Can you work these out from the drawing? Everything is in mm from the part's minimum corner. A direction names the side the tool comes from. Round coordinates to 2 decimals unless told otherwise and drop trailing zeros. Loops run counter-clockwise (first coordinate to the right, second up) from the corner with the lowest first, then second, coordinate; pieces in that order, holes last. Notation, with made-up numbers: (21.25, 18) -> (58.25, 18) arc R32 cw to (58.25, 55) -> close; hole circle Ø11 at (17.25, -13.75). An arc over 180 degrees is marked (long way). One line per item, written item: value.
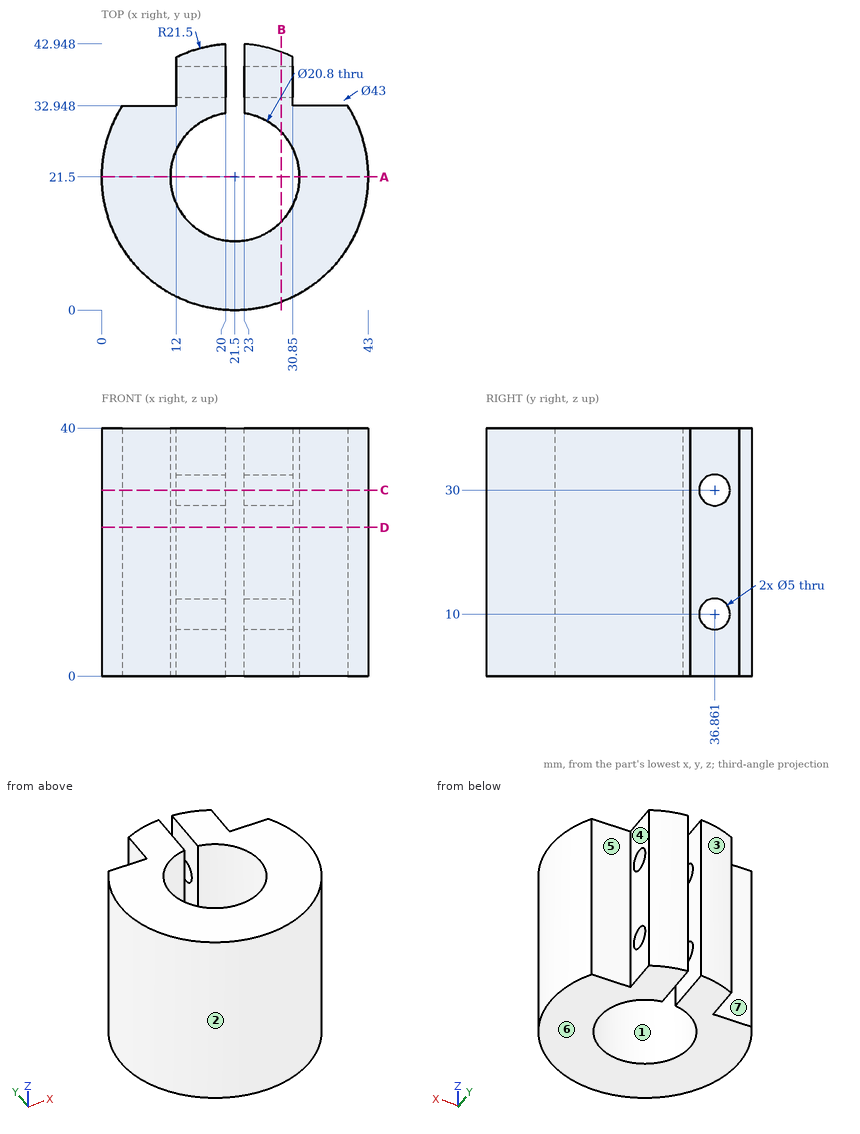
(1) For pin 1 Ø12 at (x, z) = (36.5, 27.5) entering from -Y (1 decimal); pin 2 Ø4.5 at (y, z) = (36.86, 30) entering from +X; pin 3 Ø2.5 at (x, z) = (35.5, 12) entering from +Y; pin 4 Ø5 at (y, z) = (25, 30.5) entering from -X, each with a flat end and sliding along its axis, tell me the tip position at first contact or that it passes through.
Results below:
pin 1: stops at y = 2
pin 2: passes through
pin 3: stops at y = 32.95
pin 4: stops at x = 0.02
(2) Imagine slicing it at A-A on y = 21.5. Write out the boundary of the cut face in (x, z), then the cut area to 3 significant figures.
Results below:
outline: (0, 0) -> (11.1, 0) -> (11.1, 40) -> (0, 40) -> close; (31.9, 0) -> (43, 0) -> (43, 40) -> (31.9, 40) -> close
area: 888 mm²
(3) Imagine slicing it at C-C on z = 30. Write out the boundary of the cut face in (x, y).
Results below:
outline: (3.3, 32.95) arc R21.5 ccw (long way) to (39.7, 32.95) -> (30.85, 32.95) -> (30.85, 34.36) -> (23, 34.36) -> (23, 31.79) arc R10.4 cw (long way) to (20, 31.79) -> (20, 34.36) -> (12, 34.36) -> (12, 32.95) -> close; (12, 39.36) -> (20, 39.36) -> (20, 42.95) arc R21.5 ccw to (12, 40.79) -> close; (23, 39.36) -> (30.85, 39.36) -> (30.85, 40.86) arc R21.5 ccw to (23, 42.95) -> close
(4) Imagine slicing it at D-D on z = 24. Write out the boundary of the cut face in (x, y).
Results below:
outline: (3.3, 32.95) arc R21.5 ccw (long way) to (39.7, 32.95) -> (30.85, 32.95) -> (30.85, 40.86) arc R21.5 ccw to (23, 42.95) -> (23, 31.79) arc R10.4 cw (long way) to (20, 31.79) -> (20, 42.95) arc R21.5 ccw to (12, 40.79) -> (12, 32.95) -> close
(5) On a 3-axis mill with a long thin cutter (end or side, diameter ignored), from which of +Z, -Z, +X, -X, +Y, -Y can I reach the whole of each face in a straight line? I mean the marked faces 5, 6 and 7. Say none if no direction works.
Results below:
face 5: +Z, -Z, +X, +Y
face 6: -Z, +X, -X, +Y, -Y
face 7: +Z, -Z, -X, +Y
(6) We'd pull the mould along Y, two halves only. Please class the marked faces 1, 2, 3 and 4: +Y half, -Y half, draft (parallel to the pull), parting line (faces both ways), or undercut.
Results below:
face 1: undercut
face 2: parting line
face 3: +Y half
face 4: draft
(7) Please list where these lines run through material, in increasing order: L1, parallel to X at y = 39.5, z = 8.5; L2, parallel to Y at x = 16.5, z = 31.5; L3, parallel to Y at x = 15.5, z = 30 (1 decimal).
Results below:
L1: x = 12 to 20, 23 to 30.85
L2: y = 0.59 to 12.38, 30.62 to 34.86, 38.86 to 42.41
L3: y = 0.9 to 13, 30 to 34.4, 39.4 to 42.1
(8) Imagine slicing it at B-B on x = 29. Give the number of separate pieces and of enclosed holes in the cut face.
Results below:
separate pieces: 2
enclosed holes: 2
